Input: part model. Units: mm. Frame: model coordinates. A direction names the side the tool comes from. Coordinates: 2 decimals unless noted, no trailing zeros. Write each loop counter-clockwise with the first axis right and the second up, starting at its lowest first coordinate (ties: lowest second). Pieces come first, ordered by that corner, then holes. Notation, with made-up numbers: (8.5, 10) -> (65.5, 10) arc R27 ccw to (65.5, 37) -> close; hole circle Ø9 at (-25.5, 31). An arc over 180 degrees is marked (long way). Use one line per item in the form item = value. Start each with the question number.
(1) First-contact query: pin 1 (3 mm diameter, centred on x = 1.5, y = 13.5, fed in from +Z); pin 2 (3.5 mm diameter, centred on x = 14.33, y = 8.28, fed in from +Z); pin 3 (3.5 mm diameter, centred on x = 14.33, y = 8.28, fed in from -Z). Flat tips, straight axial feed; report the tip coordinate or a pass-through.
(2) Pull-direction query (X, two-part tool) for faces 1 (the face through (19, 1.2, 10.3)), 2 (the face through (8.414, 2.758, -8.374)), 3 (the face through (17, -2, 0)); classes: released by +X, released by -X, zero draft, split by the parting line, or undercut.
(3) Cut plane A-A on x = 25. Return the cut outline in (y, z), plus the area to 3 significant figures.
(4) Ray query, line 1 along Z through (x, y) = (8.5, 5); line 2 along Y through (x, z) = (13.5, -7); line 3 along Y through (x, z) = (13, -6.5). Return the intervals inside material, ascending.
(5) Cut plane C-C on x = 9.5. State how many separate pieces and enclosed holes the cut face has, plus the area to 3 significant figures.
(6) Set-up query: faces 4 (the face through (33.3, -4.48, -2.19)), 5 (the face through (10, 2, -10.1)), 6 (the face through (13.068, 9.081, 7.671)), 7 (the face through (14.78, 10.58, -8.37)), 8 (the face through (23, -3, -6)). Return all of +Z, -Z, +X, -X, +Y, -Y with unobstructed straight access to the full face (end or side cutting, diameter ignored); none if empty.
(7) Cut plane B-B on y = -4.25. Return the cut outline in (x, z), plus the area to 3 significant figures.
```python
from build123d import *

# Parameters (mm, degrees)
SKETCH2_W           = 21.7
SKETCH2_H           = 25.05
SKETCH2_RX          = 9.525
SKETCH2_RY          = 6.35
BOSS_EXTRUDE1_DEPTH = 12.7
SKETCH3_W           = 21.660653916
SKETCH3_H           = 25.05
BOSS_EXTRUDE2_DEPTH = 3
SKETCH5_W           = 18.892037138
SKETCH5_H           = 21.7
BOSS_EXTRUDE3_DEPTH = 2
SKETCH6_W           = 30
SKETCH6_H           = 21.7
BOSS_EXTRUDE4_DEPTH = 4
SKETCH7_W           = 21.7
SKETCH7_H           = 1
SKETCH7_W_2         = 3.175
SKETCH7_H_2         = 3
CUT_EXTRUDE2_DEPTH  = 23
SKETCH7_3_W         = 21.7
SKETCH7_3_H         = 7.272473706
CUT_EXTRUDE3_DEPTH  = 44.803879418
SKETCH11_R          = 1
CUT_EXTRUDE8_DEPTH  = 33.487034031
SKETCH15_W          = 4
SKETCH15_H          = 3.5
CUT_EXTRUDE9_DEPTH  = 28.443249292
CUT_EXTRUDE4_REACH  = 47.088
SKETCH9_R           = 1.5
SKETCH10_R          = 2
CUT_EXTRUDE7_DEPTH  = 1
FILLET5_R           = 6.35
FILLET6_R           = 2
FILLET7_R           = 2


with BuildPart() as part:
    # Sketch2 → Boss-Extrude1 (new body)
    with BuildSketch(Plane(origin=(16.497783942, 9.525, 0), x_dir=(0, 0, -1), z_dir=(0.8660254037844379, 0.5000000000000013, 0))):
        Rectangle(SKETCH2_W, SKETCH2_H)
        with Locations(Location((0, 0), (0, 0, 90))):
            Ellipse(SKETCH2_RX, SKETCH2_RY, mode=Mode.SUBTRACT)
    extrude(amount=-BOSS_EXTRUDE1_DEPTH)

    # Sketch3 → Boss-Extrude2 (add)
    with BuildSketch(Plane(origin=(5.499261314, 3.175, 0), x_dir=(0, 0, 1), z_dir=(-0.8660254037844379, -0.5000000000000014, 0))):
        with Locations((-0.019673042, 0)):
            Rectangle(SKETCH3_W, SKETCH3_H)
    extrude(amount=BOSS_EXTRUDE2_DEPTH)

    # Sketch5 → Boss-Extrude3 (add)
    with BuildSketch(Plane(origin=(0, 0, 0), x_dir=(-1, 0, 0), z_dir=(0, 1, 0))):
        with Locations((-13.314265373, 0)):
            Rectangle(SKETCH5_W, SKETCH5_H)
    extrude(amount=-BOSS_EXTRUDE3_DEPTH)

    # Sketch6 → Boss-Extrude4 (add)
    with BuildSketch(Plane.XZ.offset(2)):
        with Locations((18.868246804, 0)):
            Rectangle(SKETCH6_W, SKETCH6_H)
    extrude(amount=BOSS_EXTRUDE4_DEPTH)

    # Sketch7 → Cut-Extrude2 (cut)
    with BuildSketch(Plane(origin=(33.868246804, 0, 0), x_dir=(0, 0, -1), z_dir=(1, 0, 0))):
        with Locations((0, -2.5)):
            Rectangle(SKETCH7_W, SKETCH7_H)
        with Locations((0, -4.5)):
            Rectangle(SKETCH7_W_2, SKETCH7_H_2)
    extrude(amount=-CUT_EXTRUDE2_DEPTH, mode=Mode.SUBTRACT)

    # Sketch7<3> → Cut-Extrude3 (cut, through all)
    with BuildSketch(Plane(origin=(33.868246804, 0, 0), x_dir=(0, 0, -1), z_dir=(1, 0, 0))):
        with Locations((0, -9.636236853)):
            Rectangle(SKETCH7_3_W, SKETCH7_3_H)
    extrude(amount=-CUT_EXTRUDE3_DEPTH, mode=Mode.SUBTRACT)

    # Sketch11 → Cut-Extrude8 (cut, through all)
    with BuildSketch(Plane(origin=(19.672783942, 0.194872981, 0), x_dir=(0, 0, -1), z_dir=(-1, 0, 0))):
        with Locations(Location((0, -3.830865705, 0), (0, 0, 90))):
            Circle(SKETCH11_R)
    extrude(amount=CUT_EXTRUDE8_DEPTH, mode=Mode.SUBTRACT)

    # Sketch15 → Cut-Extrude9 (cut, symmetric)
    with BuildSketch(Plane(origin=(16.497783942, 9.525, 0), x_dir=(0.7757354378747654, -0.6310582623064579, 0), z_dir=(0.6310582623064579, 0.7757354378747654, 0))):
        with Locations((0, -8.35)):
            Rectangle(SKETCH15_W, SKETCH15_H)
    cut_extrude9 = extrude(amount=CUT_EXTRUDE9_DEPTH, both=True, mode=Mode.SUBTRACT)

    # Sketch9 → Cut-Extrude4 (cut, up to next)
    with BuildSketch(Plane(origin=(0, 0, -10.85), x_dir=(-1, 0, 0), z_dir=(0, 0, -1)), mode=Mode.PRIVATE) as cut_extrude4_sk1:
        with Locations((-14.332720433, 8.275)):
            Circle(SKETCH9_R)
    cut_extrude4_tool1 = extrude(cut_extrude4_sk1.sketch, amount=-CUT_EXTRUDE4_REACH, mode=Mode.PRIVATE) & part.part
    cut_extrude4 = cut_extrude4_tool1.solids().sort_by_distance((14.33272, 8.275, -10.85))[0]
    add(cut_extrude4, mode=Mode.SUBTRACT)

    # Sketch10 → Cut-Extrude7 (cut)
    with BuildSketch(Plane(origin=(0, 0, -10.85), x_dir=(-1, 0, 0), z_dir=(0, 0, -1))):
        with Locations((-14.332720433, 8.275)):
            Circle(SKETCH10_R)
    cut_extrude7 = extrude(amount=-CUT_EXTRUDE7_DEPTH, mode=Mode.SUBTRACT)

    # Mirror1: Cut-Extrude9, Cut-Extrude4, Cut-Extrude7 across plane
    add(cut_extrude9.mirror(Plane.XY), mode=Mode.SUBTRACT)
    add(cut_extrude4.mirror(Plane.XY), mode=Mode.SUBTRACT)
    add(cut_extrude7.mirror(Plane.XY), mode=Mode.SUBTRACT)

    # Fillet5
    fillet5_edges = [part.edges().sort_by_distance(p)[0] for p in [
        (33.868246804, -4.5, 10.85),
        (33.868246804, -4.5, -10.85),
        (22.760283942, -1, -10.85),
        (22.760283942, -1, 10.85),
        (4.736022628, 17.196968182, 10.85),
        (3.436984522, 16.446968182, -10.85),
    ]]
    fillet(fillet5_edges, radius=FILLET5_R)

    # Fillet6
    fillet6_edges = [part.edges().sort_by_distance(p)[0] for p in [
        (33.868246804, -4.5, 1.5875),
        (33.868246804, -4.5, -1.5875),
    ]]
    fillet(fillet6_edges, radius=FILLET6_R)

    # Fillet7
    # the kernel refuses this fillet: 2 mm, written as the material it takes off along each edge
    with BuildSketch(Plane(origin=(22.760283942, 0, 8.429393602), x_dir=(-1, 0, 0), z_dir=(0, 0, -1))) as fillet7_piece_1:
        with BuildLine():
            CenterArc((2, -1.571757441), FILLET7_R, 128.197977663, 51.802022337)
            Line((0, -1.571757441), (-0.04, -1.571757441))
            Line((-0.04, -1.571757441), (-0.04, 0))
            Line((-0.04, 0), (0, 0.04))
            ThreePointArc((0, 0.04), (0.381619343, 0.04), (0.73850346, 0.031435149))
            Line((0.73850346, 0.031435149), (0.763238686, 0))
        make_face()
    extrude(amount=16.858787203, mode=Mode.SUBTRACT)


solid = part.part
```
Values:
q1.pin_1 = 9.95
q1.pin_2 = 9.85
q1.pin_3 = -9.85
q2.face_1 = released by +X
q2.face_2 = undercut
q2.face_3 = zero draft
q3.outline = (-6, -10.85) -> (-3, -10.85) -> (-3, -1.59) -> (-6, -1.59) -> close; (-6, 1.59) -> (-3, 1.59) -> (-3, 10.85) -> (-6, 10.85) -> close
q3.area = 55.6 mm2
q4.line_1 = -10.85 to -6.35, 6.35 to 10.85
q4.line_2 = -6 to -3, -2 to 2.67, 9.52 to 14.72
q4.line_3 = -6 to -3, -2 to 7.59, 8.96 to 15.58
q5.separate_pieces = 1
q5.enclosed_holes = 3
q5.area = 322 mm2
q6.face_4 = +X, +Y, -Y
q6.face_5 = none
q6.face_6 = +Z, -Z
q6.face_7 = +X
q6.face_8 = +Z, -Z, +X
q7.outline = (3.87, -10.85) -> (27.52, -10.85) arc R6.35 ccw to (33.87, -4.5) -> (33.87, -3.59) arc R2 ccw to (31.87, -1.59) -> (10.87, -1.59) -> (10.87, 1.59) -> (31.87, 1.59) arc R2 ccw to (33.87, 3.59) -> (33.87, 4.5) arc R6.35 ccw to (27.52, 10.85) -> (3.87, 10.85) -> (3.87, 10.1) -> (7.87, 10.1) -> (7.87, 6.6) -> (3.87, 6.6) -> (3.87, -6.6) -> (7.87, -6.6) -> (7.87, -10.1) -> (3.87, -10.1) -> close
q7.area = 531 mm2
